Build history of the part. All positions in model axes, mm. A direction names the side the tool comes from. Coordinates: 2 decimals unless noted, no trailing zeros. Write each loop counter-clockwise with the first axis right and the second up, starting at its lowest first coordinate (ties: lowest second). Pieces come first, ordered by that corner, then holes.
```python
from build123d import *

# Parameters (mm, degrees)
F0_W     = 34
F0_H     = 198
F1_DEPTH = 25
F2_DEPTH = 0.2
F3_W     = 20
F3_H     = 184
F4_DEPTH = 25
F6_DEPTH = 0.2


with BuildPart() as f1:
    # F0 (on Front) → F1 (new body)
    with BuildSketch(Plane.XZ):
        Rectangle(F0_W, F0_H)
    extrude(amount=F1_DEPTH)

    # F0 (on Front) → F2 (join)
    with BuildSketch(Plane.XZ):
        Rectangle(F0_W, F0_H)
    extrude(amount=-F2_DEPTH)

    # F3 (on face) → F4 (cut)
    with BuildSketch(Plane.XZ.offset(25)):
        Rectangle(F3_W, F3_H)
    extrude(amount=-F4_DEPTH, mode=Mode.SUBTRACT)

    # F5 (on face) → F6 (join)
    with BuildSketch(Plane.XZ.offset(25)):
        Polygon((17, 99), (-17, 99), (-10, 92), (10, 92), align=None)
        Polygon((-10, -92), (-17, -99), (17, -99), (10, -92), align=None)
    extrude(amount=F6_DEPTH)


solid = f1.part
```
1. Saw through at C-C on z = 67. List the corners of the cut face in (x, y), plus the area to 3 significant figures.
Computed values:
outline: (-17, -25) - (-10, -25) - (-10, 0) - (10, 0) - (10, -25) - (17, -25) - (17, 0.2) - (-17, 0.2) - close
area: 357 mm2
2. Mould opens along X. For faces 3 (the face through (0, -12, 92)), 4 (the face through (17, -13, -1)), 5 (the face through (0, 0.2, 1)) say: +X half, -X half, draft (parallel to the pull), parting line (faces both ways), or undercut.
Computed values:
face 3: undercut
face 4: +X half
face 5: draft
3. Saw through at A-A on y = -2.25. List the corners of the cut face in (x, z), plus the area to 3 significant figures.
Computed values:
outline: (-17, -99) - (17, -99) - (17, 99) - (-17, 99) - close; hole (-10, -92) - (10, -92) - (10, 92) - (-10, 92) - close
area: 3,050 mm2
4. Probe line 1 along X through (y, z) = (-12.75, 75.5); line 2 along Z through (x, y) = (-6, -9.5); line 3 along Y through (x, z) = (-15, 21.5). List the from-to ranges inside material, lowest first.
Computed values:
line 1: x = -17 to -10, 10 to 17
line 2: z = -99 to -92, 92 to 99
line 3: y = -25 to 0.2
5. Flat gauge pins, fed straight in: pin 1 (4 mm diameter, centred on x = 8.5, z = -8.5, fed in from -Y); pin 2 (10 mm diameter, centred on x = 2.5, z = -6, fed in from -Y). Where does each tip first touch, or does it go through?
Computed values:
pin 1: stops at y = -25
pin 2: stops at y = 0
6. 3-axis set-ups, long thin cutter, end or side, ignore diameter. For faces 1 (the face through (0, -13, -99)), 2 (the face through (0, -12, -92)): which of +Z, -Z, +X, -X, +Y, -Y reach the whole face in a straight line?
Computed values:
face 1: -Z, +X, -X, +Y, -Y
face 2: -Y
7. Saw through at B-B on x = 7. List the corners of the cut face in (y, z).
Computed values:
outline: (-25.2, -99) - (0.2, -99) - (0.2, 99) - (-25.2, 99) - (-25.2, 92) - (0, 92) - (0, -92) - (-25.2, -92) - close
